For this review, take the finished solid that the model builds, in its own axes (mm). A direction names the side the tool comes from. Round coordinates to 2 decimals unless told otherwise and drop trailing zeros. Loops run counter-clockwise (first coordinate to the right, second up) from the corner with the lowest first, then second, coordinate; pieces in that order, holes last. Notation, with made-up numbers: (66.25, 57) -> (95.25, 57) arc R27 cw to (95.25, 92) -> close; hole circle Ø11 at (49.5, 16.25). An arc over 180 degrees is marked (long way). One line per question, with ' | ' between items. Start each with the question number.
1. Wall thickness on line 1 along Y through (x, z) = (4.75, 3); line 2 along Y through (x, z) = (4.25, 0.25); line 3 along Z through (x, y) = (2.5, 1.5): over which ranges is each line inside the solid? List them lowest first.
2. For faces 1 (the face through (3, -10.016, 2)), 2 (the face through (3, -26.67, 0)), list the 3-axis set-ups (+Z, -Z, +X, -X, +Y, -Y) from which the entire face can be reached by the end or side of a thin tool; tool diameter is ignored.
3. Consider section A-A (x = 1). Write out the cut boundary in (y, z).
4. Consider section B-B (z = 2.75). Write out the cut boundary in (x, y), and give its area (3 significant figures).
5. Consider section D-D (z = 0.5). Write out the cut boundary in (x, y).
6. Draft analysis for pull direction Z (two halves, no side actions). For faces 3 (the face through (3, -3.666, 2)), 4 (the face through (3, -11, -3.81)), 5 (the face through (3.13, 1.26, 0.17)), state which applies: pulls with the +Z half, pulls with the -Z half, needs draft (parallel to the pull), parting line crosses it, or undercut.
7. For pin 1 Ø1.9 at (x, y) = (4, -8.5) entering from +Z; pin 2 Ø0.8 at (x, z) = (4.5, 2.5) entering from +Y, all flat-tipped, find the tip position at first contact; note any pin that passes through.
8. Consider section C-C (y = -9.5). Write out the cut boundary in (x, z), and give its area (3 significant figures).
```python
from build123d import *

# Parameters (mm, degrees)
ELEVATOR_PADDLE_R   = 1.27
BOSS_EXTRUDE1_DEPTH = 6.35


with BuildPart() as part:
    # Elevator Paddle → Boss-Extrude1 (new body)
    with BuildSketch(Plane(origin=(0, 0, 0), x_dir=(0, 0, -1), z_dir=(1, 0, 0))):
        with BuildLine():
            Line((3.81, 3.81), (3.81, -26.67))
            Line((3.81, -26.67), (-3.81, -26.67))
            Line((-3.81, -26.67), (-3.81, -10.0160188))
            Line((-3.81, -10.0160188), (-1.037499957, -10.0160188))
            Line((-1.037499957, -10.0160188), (-1.037499957, -3.6660188))
            Line((-1.037499957, -3.6660188), (-3.81, -3.6660188))
            Line((-3.81, -3.6660188), (-3.81, 0))
            ThreePointArc((-3.81, 0), (-2.694076836, 2.694076836), (0, 3.81))
            Line((0, 3.81), (3.81, 3.81))
        make_face()
        Circle(ELEVATOR_PADDLE_R, mode=Mode.SUBTRACT)
    extrude(amount=BOSS_EXTRUDE1_DEPTH)


solid = part.part
```
Answer block:
1) line 1: y = -26.67 to -10.02, -3.67 to 2.35 | line 2: y = -26.67 to -1.25, 1.25 to 3.8 | line 3: z = -3.81 to 3.5
2) face 1: +Z, +X, -X | face 2: +Z, -Z, +X, -X, -Y
3) outline: (-26.67, -3.81) -> (3.81, -3.81) -> (3.81, 0) arc R3.81 ccw to (0, 3.81) -> (-3.67, 3.81) -> (-3.67, 1.04) -> (-10.02, 1.04) -> (-10.02, 3.81) -> (-26.67, 3.81) -> close; hole circle Ø2.54 at (0, 0)
4) outline: (0, -26.67) -> (6.35, -26.67) -> (6.35, -10.02) -> (0, -10.02) -> close; (0, -3.67) -> (6.35, -3.67) -> (6.35, 2.64) -> (0, 2.64) -> close | area: 146 mm2
5) outline: (0, -26.67) -> (6.35, -26.67) -> (6.35, -1.17) -> (0, -1.17) -> close; (0, 1.17) -> (6.35, 1.17) -> (6.35, 3.78) -> (0, 3.78) -> close
6) face 3: needs draft | face 4: pulls with the -Z half | face 5: undercut
7) pin 1: stops at z = 1.04 | pin 2: stops at y = 3.18
8) outline: (0, -3.81) -> (6.35, -3.81) -> (6.35, 1.04) -> (0, 1.04) -> close | area: 30.8 mm2
